Work out the finished part from the listing and answer in its coordinate system (mm). A direction names the side the tool comes from. Round coordinates to 2 decimals unless told otherwise and drop trailing zeros. Loops run counter-clockwise (first coordinate to the right, second up) from the corner with the lowest first, then second, coordinate; pieces in that order, holes last. Notation, with made-up numbers: (-37, 76.25) -> (-32, 76.25) arc R11 ccw to (-32, 95.25) -> close; hole circle Ø1 at (58.25, -11). An arc over 180 degrees is marked (long way). Write item = value, one per line. Start each with the question number.
Autodesk Inventor part; units mm, degrees
ref_plane "YZ Plane" through (0, 0, 0) normal (1, 0, 0) x (0, 1, 0)
ref_plane "XZ Plane" through (0, 0, 0) normal (0, 1, 0) x (-1, 0, 0)
ref_plane "XY Plane" through (0, 0, 0) normal (0, 0, 1) x (1, 0, 0)
sketch "Sketch1" plane through (0, 0, 0) normal (0, 1, 0) x (-1, 0, 0)
  line L0 (0, -6) -> (0, 0)
  line L1 (0, 0) -> (-12, 0)
  line L2 (-12, 0) -> (-12, 13)
  line L3 (-12, 13) -> (0, 13)
  line L4 (0, 13) -> (0, 67)
  line L5 (0, 67) -> (-8, 75)
  line L6 (-8, 75) -> (-67, 75)
  line L7 (-67, 75) -> (-75, 67)
  line L8 (0, -6) -> (-100, -50)
  line L9 (-100, -50) -> (-124.5, -50)
  line L10 (-124.5, -50) -> (-124.5, 0)
  line L11 (-124.5, 0) -> (-118.5, 0)
  line L12 (-118.5, 0) -> (-118.5, 13)
  line L13 (-118.5, 13) -> (-124.5, 13)
  line L14 (-124.5, 13) -> (-124.5, 19)
  line L15 (-124.5, 19) -> (-75, 19)
  line L16 (-75, 19) -> (-75, 67)
  circle A0 centre (-26, 55) radius 4
  circle A1 centre (-49, 55) radius 2.5
  line L17 (-106, -50) -> (-112.5, -50) construction
  line L18 (-112.5, -50) -> (-112.5, 13) construction
  line L19 (-112.5, 13) -> (-106, 13) construction
  line L20 (-106, 13) -> (-106, -50) construction
  dimension "d0" = 13
  dimension "d1" = 12
  dimension "d2" = 6
  dimension "d3" = 6
  dimension "d4" = 6
  dimension "d6" = 75
  dimension "d7" = 8
  dimension "d8" = 5
  dimension "d9" = 23
  dimension "d10" = 106.5
  dimension "d11" = 45
  dimension "d12" = 8
  dimension "d13" = 6.5
  dimension "d14" = 6
  dimension "d15" = 6
  dimension "d16" = 42
  dimension "d17" = 20
  dimension "d18" = 50
  dimension "d19" = 26
extrude "Extrusion1" add sketch "Sketch1" along normal blind 6.5
sketch "Sketch3" plane through (0, 6.5, 0) normal (0, 1, 0) x (1, 0, 0)
  line L0 (124.5, 0) -> (124.5, 50)
  line L1 (124.5, 50) -> (100, 50)
  line L2 (106, 50) -> (112.5, 50)
  line L3 (112.5, 50) -> (112.5, 44)
  line L4 (112.5, 44) -> (106, 44)
  line L5 (106, 44) -> (106, 50)
  dimension "d27" = 6
  dimension "d28" = 6.5
  dimension "d29" = 12
extrude "Extrusion3" cut sketch "Sketch3" against normal through all
chamfer "Chamfer1" distance 2 angle 45 3 edges at (75, 3.25, 19) (124.5, 3.25, 19) (124.5, 3.25, -50)
sketch "Sketch4" plane through (0, 6.5, 0) normal (0, 1, 0) x (1, 0, 0)
  line L0 (124.5, 0) -> (124.5, 48)
  circle A0 centre (26, -55) radius 4
  circle A1 centre (49, -55) radius 2.5
  circle A2 centre (37.5, -47.5) radius 2.25
  circle A3 centre (37.5, -62.5) radius 2.25
  line L1 (37.5, -47.5) -> (37.5, -62.5) construction
  line L2 (26, -55) -> (49, -55) construction
  point P0 (37.5, -55)
  dimension "d35" = 15
  dimension "d36" = 4.5
extrude "Extrusion4" cut sketch "Sketch4" against normal through all contours A2 | A3
sketch "Sketch5" plane through (0, 6.5, 0) normal (0, 1, 0) x (1, 0, 0)
  line L0 (112.5, 44) -> (106, 44)
  line L1 (12, 0) -> (12, -13)
  line L2 (0, -13) -> (0, -67)
  line L3 (118.5, -13) -> (118.5, 0)
  line L4 (118.5, 0) -> (124.5, 0)
  circle A0 centre (22.217, -6.5) radius 2.25
  circle A1 centre (93.5, -6.5) radius 2.25
  circle A2 centre (109.25, 28) radius 2.25
  point P0 (12, -6.5)
  point P1 (109.25, 44)
  dimension "d39" = 4.5
  dimension "d40" = 22.217
  dimension "d41" = 25
  dimension "d42" = 28
extrude "Extrusion5" cut sketch "Sketch5" against normal through all
equation "\"d2\" = d3"
equation "\"d4\" = d3"
properties part number "z_axis_top"
Item 1: Flat-ended cylindrical pins translate along their axes: pin 1 (1.8 mm diameter, centred on x = 122, y = 3.5, fed in from +Z); pin 2 (2 mm diameter, centred on x = 19, y = 6, fed in from -Z); pin 3 (3 mm diameter, centred on x = 109, y = 3, fed in from -Z). Find the tip coordinate at first contact, or state that the pin passes through.
Item 2: Section C-C (y = 5.5) is taken. Count the separate pieces of the cut face and the enclosed holes in it, then the cut area to 3 significant figures.
Item 3: Section D-D (z = 55) is taken. Determine the outline of the cut face in (x, y).
Item 4: Section A-A (z = 6.5) is taken. Determine the outline of the cut face in (x, y).
Item 5: Find the intervals of material crossed by line 1 along X through (y, z) = (3.75, 6.5); line 2 along Z through (x, y) = (109.25, 3.5); line 3 along Z through (x, y) = (37.5, 3.25), in increasing order. Write a range as [from, to].
Item 6: The mould has two halves that part along X. Classify faces 1 (the flat face through (118.5, 3, 6)), 2 (the cylindrical face through (23.427, 3.296, 4.603)), 3 (the flat face through (103, 3, -50)), 4 (the cylindrical face through (26.867, 3.204, 58.905)): pulls with the +X half, pulls with the -X half, needs draft (parallel to the pull), parting line crosses it, or undercut.
Item 7: Section B-B (x = 49) is taken. Determine the outline of the cut face in (y, z).
Item 8: A tool of negligible diameter and unlimited length cuts with its end or side. For faces 5 (the flat face through (6, 3, 0)), 6 (the flat face through (100, 3, 19)), 7 (the flat face through (121, 3, 13)), from which of +Z, -Z, +X, -X, +Y, -Y can it reach the whole face along a straight path? Write none if from no direction.
Worked answers:
q1.pin_1 = 19
q1.pin_2 = -14.8
q1.pin_3 = -44
q2.separate_pieces = 1
q2.enclosed_holes = 7
q2.area = 10,100 mm2
q3.outline = (0, 0) -> (22, 0) -> (22, 6.5) -> (0, 6.5) -> close; (30, 0) -> (46.5, 0) -> (46.5, 6.5) -> (30, 6.5) -> close; (51.5, 0) -> (75, 0) -> (75, 6.5) -> (51.5, 6.5) -> close
q4.outline = (12, 0) -> (19.97, 0) -> (19.97, 6.5) -> (12, 6.5) -> close; (24.47, 0) -> (91.25, 0) -> (91.25, 6.5) -> (24.47, 6.5) -> close; (95.75, 0) -> (118.5, 0) -> (118.5, 6.5) -> (95.75, 6.5) -> close
q5.line_1 = [12, 19.97], [24.47, 91.25], [95.75, 118.5]
q5.line_2 = [-44, -30.25], [-25.75, 19]
q5.line_3 = [-22.5, 45.25], [49.75, 60.25], [64.75, 75]
q6.face_1 = pulls with the +X half
q6.face_2 = undercut
q6.face_3 = needs draft
q6.face_4 = undercut
q7.outline = (0, -27.56) -> (6.5, -27.56) -> (6.5, 52.5) -> (0, 52.5) -> close; (0, 57.5) -> (6.5, 57.5) -> (6.5, 75) -> (0, 75) -> close
q8.face_5 = -X, +Y, -Y
q8.face_6 = +Z, +X, +Y, -Y
q8.face_7 = +X, +Y, -Y
